Job drawing, mm, ordinate dimensions from the low corner. One solid piece. A direction names the side the tool comes from. Round coordinates to 2 decimals unless told otherwise and drop trailing zeros. Loops run counter-clockwise (first coordinate to the right, second up) from the corner with the lowest first, then second, coordinate; pieces in that order, holes last. Notation, with made-up numbers: M 56,-32.75 L 83,-32.75 A9 cw 83,-21.75 Z; hole C 5.5,41.25 d11. An arc over 180 degrees is marked long. Put each result on its own line as item: value. Start each with the question number.
1) Probe line 1 along Y through (x, z) = (14.6, 7.5) (1 decimal); line 2 along X through (y, z) = (10.5, 17); line 3 along X through (y, z) = (4, 9.5). List the from-to ranges inside material, lowest first.
2) Drop flat-ended pins along their axis: pin 1 Ø12 at (y, z) = (7, 13.5) entering from +X; pin 2 Ø1.5 at (x, z) = (9, 13.5) entering from +Y (3 decimals); pin 3 Ø12 at (x, y) = (19, 7) entering from +Z; pin 4 Ø4 at (y, z) = (19.79, 7.5) entering from -X. Give the stop position or say it passes through.
3) Slice it at B-B on y = 20. Give the cut face in (x, z).
4) Slice it at D-D on z = 7.5. Give the cut face in (x, y), then the cut area to 3 significant figures.
5) Slice it at A-A on z = 20.5. Give the cut face in (x, y), then the cut area to 3 significant figures.
6) Slice it at C-C on x = 18.25. Give the cut face in (y, z).
7) Which spindle directions (+Z, -Z, +X, -X, +Y, -Y) get a long thin tool onto all of the face, cutting with end or side? Do the marked faces 1, 2 and 3. Say none if no direction does.
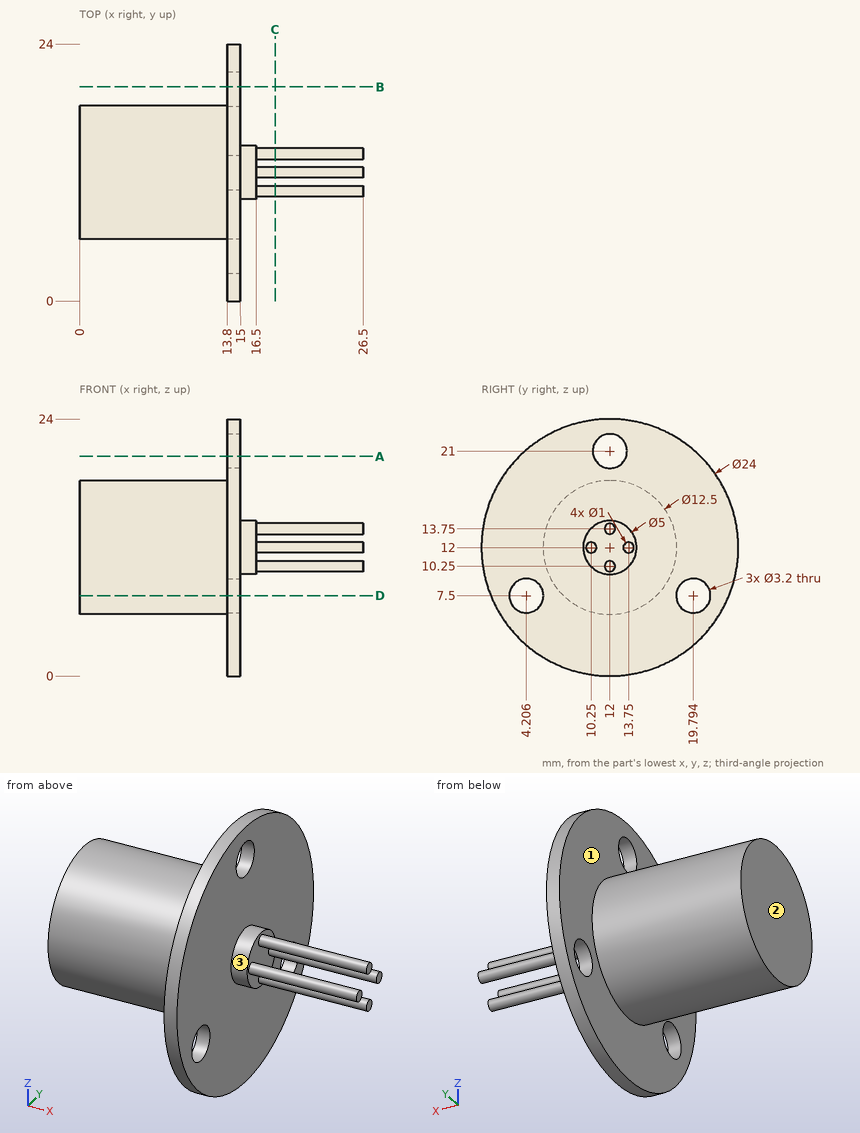
Recorded:
1. line 1: y = 0.9 to 2.6, 5.8 to 18.2, 21.4 to 23.1
1. line 2: x = 0 to 15
1. line 3: x = 13.8 to 15
2. pin 1: stops at x = 26.5
2. pin 2: stops at y = 18.205
2. pin 3: stops at z = 23.99
2. pin 4: stops at x = 13.8
3. outline: M 13.8,3.06 L 15,3.06 L 15,5.91 L 13.8,5.91 Z; M 13.8,9.09 L 15,9.09 L 15,20.94 L 13.8,20.94 Z
4. outline: M 0,7.66 L 13.8,7.66 L 13.8,5.81 L 15,5.81 L 15,18.19 L 13.8,18.19 L 13.8,16.34 L 0,16.34 Z; M 13.8,0.88 L 15,0.88 L 15,2.61 L 13.8,2.61 Z; M 13.8,21.39 L 15,21.39 L 15,23.12 L 13.8,23.12 Z
4. area: 139 mm2
5. outline: M 13.8,3.53 L 15,3.53 L 15,10.48 L 13.8,10.48 Z; M 13.8,13.52 L 15,13.52 L 15,20.47 L 13.8,20.47 Z
5. area: 16.7 mm2
6. outline: C 10.25,12 d1; C 12,10.25 d1; C 12,13.75 d1; C 13.75,12 d1
7. face 1: -X
7. face 2: +Z, -Z, -X, +Y, -Y
7. face 3: +X
